Verification items for this drawing (mm, ordinates from the low corner). A direction names the side the tool comes from. Coordinates: 2 decimals unless noted, no trailing zeros. Order: outer loops, then holes, each group sorted by start corner. A loop starts at its lowest first (then second) coordinate and runs counter-clockwise, first axis right, second up. Notation, with made-up numbers: (46.25, 71) -> (99.25, 71) arc R12 cw to (99.25, 84) -> close; hole circle Ø2 at (22, -18.75). An arc over 180 degrees is marked (long way). Answer in a Markdown table with one row per item. Add a question column.
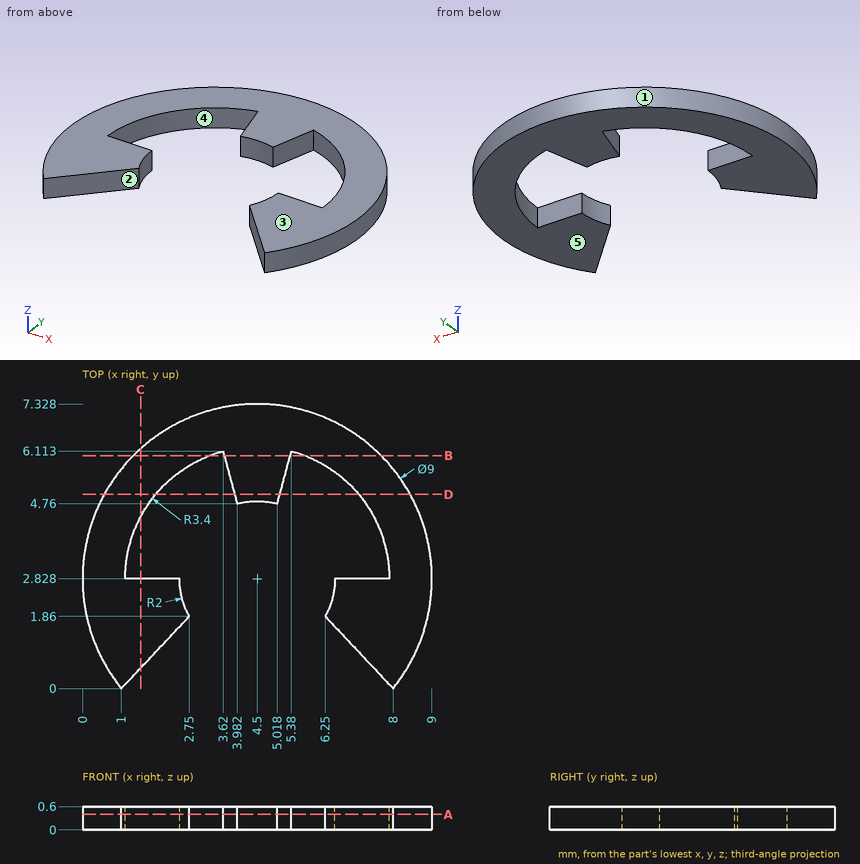
(1) Access from +Z, -Z, +X, -X, +Y, -Y to the whole of each face (thin tool, end or side, straight path). Record for the marked faces 4 and 5.
(2) Cross-section at A-A (z = 0.4). Enter the section's corners in (x, y).
(3) Cross-section at D-D (y = 5). Enter the section's corners in (x, z).
(4) Mould release check, pull along X, two halves, no side actions. Record for the marked faces 1, 2 and 3: +X half, -X half, draft (parallel to the pull), parting line (faces both ways), or undercut.
(5) Scan lines: line 1 along X through (y, z) = (5, 0.3) (1 decimal); line 2 along X through (y, z) = (3.5, 0.4); line 3 along X through (y, z) = (2.25, 0.3) (1 decimal). Record each from-to range of solid material in increasing order.
(6) Cross-section at C-C (x = 1.5). Enter the section's corners in (y, z).
(7) Cross-section at B-B (y = 6). Give the number of separate pieces and of enclosed holes in the cut face.
Checks:
| question | item | result |
|---|---|---|
| 1 | face 4 | +Z, -Z |
| 1 | face 5 | -Z, +X, -X, +Y, -Y |
| 2 | outline | (1, 0) -> (2.75, 1.86) arc R2 cw to (2.5, 2.83) -> (1.1, 2.83) arc R3.4 cw to (3.62, 6.11) -> (3.98, 4.76) arc R2 cw to (5.02, 4.76) -> (5.38, 6.11) arc R3.4 cw to (7.9, 2.83) -> (6.5, 2.83) arc R2 cw to (6.25, 1.86) -> (8, 0) arc R4.5 ccw (long way) to start |
| 3 | outline | (0.56, 0) -> (1.88, 0) -> (1.88, 0.6) -> (0.56, 0.6) -> close; (3.92, 0) -> (5.08, 0) -> (5.08, 0.6) -> (3.92, 0.6) -> close; (7.12, 0) -> (8.44, 0) -> (8.44, 0.6) -> (7.12, 0.6) -> close |
| 4 | face 1 | parting line |
| 4 | face 2 | undercut |
| 4 | face 3 | draft |
| 5 | line 1 | 0.6 to 1.9, 3.9 to 5.1, 7.1 to 8.4 |
| 5 | line 2 | 0.05 to 1.17, 7.83 to 8.95 |
| 5 | line 3 | 0 to 2.6, 6.4 to 9 |
| 6 | outline | (0.53, 0) -> (2.83, 0) -> (2.83, 0.6) -> (0.53, 0.6) -> close; (4.43, 0) -> (6.18, 0) -> (6.18, 0.6) -> (4.43, 0.6) -> close |
| 7 | separate pieces | 3 |
| 7 | enclosed holes | 0 |
